Geometry check sheet. Reference: drawing and pictorial views, mm from the part's lowest x, y, z. A direction names the side the tool comes from. Round coordinates to 2 decimals unless told otherwise and drop trailing zeros. Order: outer loops, then holes, each group sorted by start corner. A loop starts at its lowest first (then second) coordinate and runs counter-clockwise, first axis right, second up.
(1) Thickness scan on probe 1 along X at (y, z) = (32, 35); probe 2 along Y at (x, z) = (117.5, 33); probe 3 along Z at (x, y) = (75, 203). Record the ranges inside material, lowest first.
(2) Sectioned sample at C-C, the plane y = 203.2. Enter the section's corners in (x, z), and give its area (3 significant figures).
(3) Sectioned sample at B-B, the plane y = 32.5. Enter the section's corners in (x, z).
(4) Sectioned sample at A-A, the plane x = 130. Enter the section's corners in (y, z).
(5) Sectioned sample at D-D, the plane z = 60.5. Enter the section's corners in (x, y), and give its area (3 significant figures).
(6) Tool access check on the marked faces 1, 2 and 3. Record the directions out of +Z, -Z, +X, -X, +Y, -Y that give a thin tool (end or side, any length) a straight path to the whole face; none if there is none.
(7) Depth check by flat-ended pin: pin 1 (15 mm diameter, centred on x = 130, y = 32.5, fed in from -Z); pin 2 (12 mm diameter, centred on x = 40, z = 36.5, fed in from +Y); pin 3 (8 mm diameter, centred on x = 45, y = 58, fed in from +Z). Enter the tip coordinate at first touch or a pass-through.
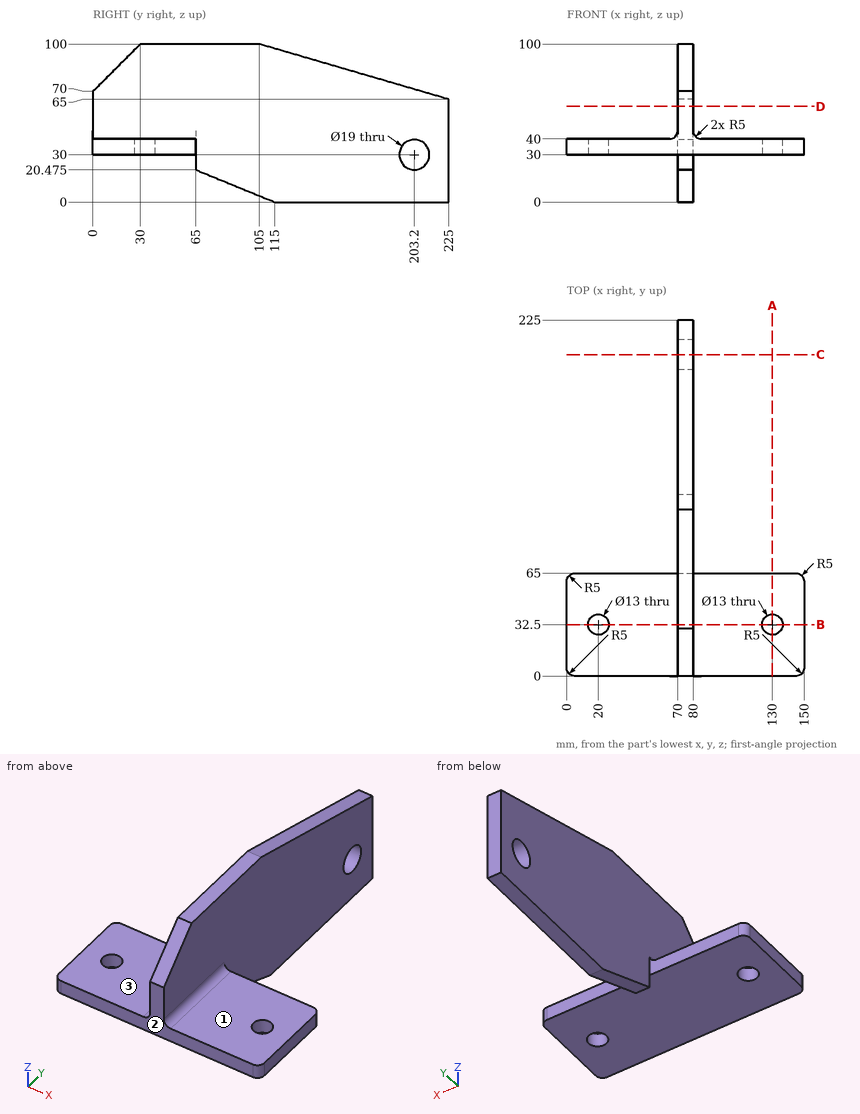
Derived:
1. probe 1: x = 0 to 13.52, 26.48 to 123.52, 136.48 to 150
1. probe 2: y = 0 to 65
1. probe 3: z = 0 to 20.5, 39.5 to 71.42
2. outline: (70, 0) - (80, 0) - (80, 20.5) - (70, 20.5) - close; (70, 39.5) - (80, 39.5) - (80, 71.36) - (70, 71.36) - close
2. area: 524 mm2
3. outline: (0, 30) - (13.5, 30) - (13.5, 40) - (0, 40) - close; (26.5, 30) - (123.5, 30) - (123.5, 40) - (85, 40) arc R5 cw to (80, 45) - (80, 100) - (70, 100) - (70, 45) arc R5 cw to (65, 40) - (26.5, 40) - close; (136.5, 30) - (150, 30) - (150, 40) - (136.5, 40) - close
4. outline: (0, 30) - (26, 30) - (26, 40) - (0, 40) - close; (39, 30) - (65, 30) - (65, 40) - (39, 40) - close
5. outline: (70, 0) - (80, 0) - (80, 225) - (70, 225) - close
5. area: 2,250 mm2
6. face 1: +Z, +X, +Y, -Y
6. face 2: +Z, -Z, +X, -X, -Y
6. face 3: +Z, -X, +Y, -Y
7. pin 1: stops at z = 30
7. pin 2: stops at y = 65
7. pin 3: stops at z = 40
